Geometry check sheet. Reference: the model listing, model coordinates, mm. Face numbers are marked on the shaded views. A direction names the side the tool comes from. Give positions to 0.01 mm unless a question says otherwise; leave off trailing zeros. Write each loop counter-clockwise with the first axis right and the second up, starting at its lowest first coordinate (ties: lowest second). Pieces come first, ordered by that corner, then holes. Notation, with made-up numbers: (-33, 50.25) -> (-9, 50.25) arc R32 ccw to (-9, 89.25) -> close; hole circle Ø4 at (-9, -38.5). An arc over 180 degrees is marked (long way). Use a Markdown table: item, result. Add a question column.
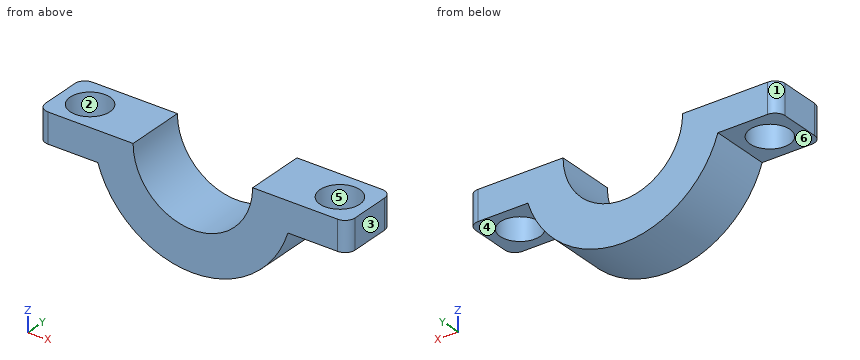
from build123d import *

# Parameters (mm, degrees)
BOSS_EXTRUDE1_DEPTH = 6
BOSS_EXTRUDE2_DEPTH = 6
SKETCH4_R           = 2
CUT_EXTRUDE2_DEPTH  = 11
FILLET1_R           = 1


with BuildPart() as part:
    # Sketch1 → Boss-Extrude1 (new body)
    with BuildSketch(Plane(origin=(0, 0, 0), x_dir=(1, 0, 0), z_dir=(0, 1, 0))):
        with BuildLine():
            Line((-10, 0), (-6, 0))
            ThreePointArc((-6, 0), (0, 6), (6, 0))
            Line((6, 0), (10, 0))
            ThreePointArc((10, 0), (0, 10), (-10, 0))
        make_face()
    extrude(amount=BOSS_EXTRUDE1_DEPTH)

    # Sketch3 → Boss-Extrude2 (add)
    with BuildSketch(Plane(origin=(0, 6, 0), x_dir=(1, 0, 0), z_dir=(0, 1, 0))):
        with BuildLine():
            Line((-10, 0), (-15.539392014, 0))
            Line((-15.539392014, 0), (-15.539392014, 3))
            Line((-15.539392014, 3), (-9.539392014, 3))
            ThreePointArc((-9.539392014, 3), (-9.884177258, 1.517576993), (-10, 0))
        make_face()
    boss_extrude2 = extrude(amount=-BOSS_EXTRUDE2_DEPTH)

    # Sketch4 → Cut-Extrude2 (cut, through all)
    with BuildSketch(Plane.XY):
        with Locations((-12.539392014, 3)):
            Circle(SKETCH4_R)
    cut_extrude2 = extrude(amount=-CUT_EXTRUDE2_DEPTH, mode=Mode.SUBTRACT)

    # Mirror2: Boss-Extrude2, Cut-Extrude2 across plane
    add(boss_extrude2.mirror(Plane(origin=(0, 0, 0), x_dir=(0, 0, 1), z_dir=(1, 0, 0))))
    add(cut_extrude2.mirror(Plane(origin=(0, 0, 0), x_dir=(0, 0, 1), z_dir=(1, 0, 0))), mode=Mode.SUBTRACT)

    # Fillet1
    fillet1_edges = [part.edges().sort_by_distance(p)[0] for p in [
        (-15.539392014, 6, -1.5),
        (-15.539392014, 0, -1.5),
        (15.539392014, 6, -1.5),
        (15.539392014, 0, -1.5),
    ]]
    fillet(fillet1_edges, radius=FILLET1_R)


solid = part.part
1) Draft check along Y on the marked faces 1, 2 and 3. Enter one of: +Y half, -Y half, draft (parallel to the pull), parting line (faces both ways), or undercut.
2) Tool access check on the marked faces 4, 5 and 6. Record the directions out of +Z, -Z, +X, -X, +Y, -Y that give a thin tool (end or side, any length) a straight path to the whole face; none if there is none.
3) Material ranges on probe 1 along Y at (x, z) = (12.5, -1); probe 2 along Y at (x, z) = (-13, -1.75); probe 3 along X at (y, z) = (0.8, -5), recorded low to high. Write a range as [from, to].
4) Sectioned sample at A-A, the plane y = 3. Enter the section's corners in (x, z), and give its area (3 significant figures).
5) Sectioned sample at C-C, the plane x = 0. Enter the section's corners in (y, z).
6) Sectioned sample at B-B, the plane z = -3.5. Enter the section's corners in (x, y).
7) Sectioned sample at D-D, the plane y = 0.4. Enter the section's corners in (x, z), and give its area (3 significant figures).
8) Gauge pin test, flat end, axial feed: P1, Ø3, axis at y = 1.5, z = -8, coming from the -X side. Record the tip position at first contact, or that the pin passes through.
Check values:
| question | item | result |
|---|---|---|
| 1 | face 1 | +Y half |
| 1 | face 2 | undercut |
| 1 | face 3 | draft |
| 2 | face 4 | -Z, +X, +Y, -Y |
| 2 | face 5 | +Z, -Z |
| 2 | face 6 | -Z, -X, +Y, -Y |
| 3 | probe 1 | [0, 1], [5, 6] |
| 3 | probe 2 | [0, 1.05], [4.95, 6] |
| 3 | probe 3 | [-8.66, -3.32], [3.32, 8.66] |
| 4 | outline | (-15.54, -3) -> (-14.54, -3) -> (-14.54, 0) -> (-15.54, 0) -> close; (-10.54, -3) -> (-9.54, -3) arc R10 ccw to (9.54, -3) -> (10.54, -3) -> (10.54, 0) -> (6, 0) arc R6 cw to (-6, 0) -> (-10.54, 0) -> close; (14.54, -3) -> (15.54, -3) -> (15.54, 0) -> (14.54, 0) -> close |
| 4 | area | 111 mm² |
| 5 | outline | (0, -10) -> (6, -10) -> (6, -6) -> (0, -6) -> close |
| 6 | outline | (-9.37, 0) -> (-4.87, 0) -> (-4.87, 6) -> (-9.37, 6) -> close; (4.87, 0) -> (9.37, 0) -> (9.37, 6) -> (4.87, 6) -> close |
| 7 | outline | (-15.34, -3) -> (-9.54, -3) arc R10 ccw to (9.54, -3) -> (15.34, -3) -> (15.34, 0) -> (6, 0) arc R6 cw to (-6, 0) -> (-15.34, 0) -> close |
| 7 | area | 133 mm² |
| 8 | P1 | x = -7.6 |
